Input: dimensioned drawing with shaded views. Units: mm. Origin: part minimum x, y, z. A direction names the side the tool comes from. Round coordinates to 2 decimals unless told otherwise and drop trailing zeros. Loops run counter-clockwise (first coordinate to the right, second up) from the corner with the lowest first, then second, coordinate; pieces in that order, holes last. Notation, with made-up numbers: (59, 1) - (102, 1) arc R29 ccw to (102, 40) - close; hole circle Ø10 at (72.5, 7). An arc over 180 degrees is marked (long way). Use CSV: the item, a comma, the result in double quotes. Start each with the question number.
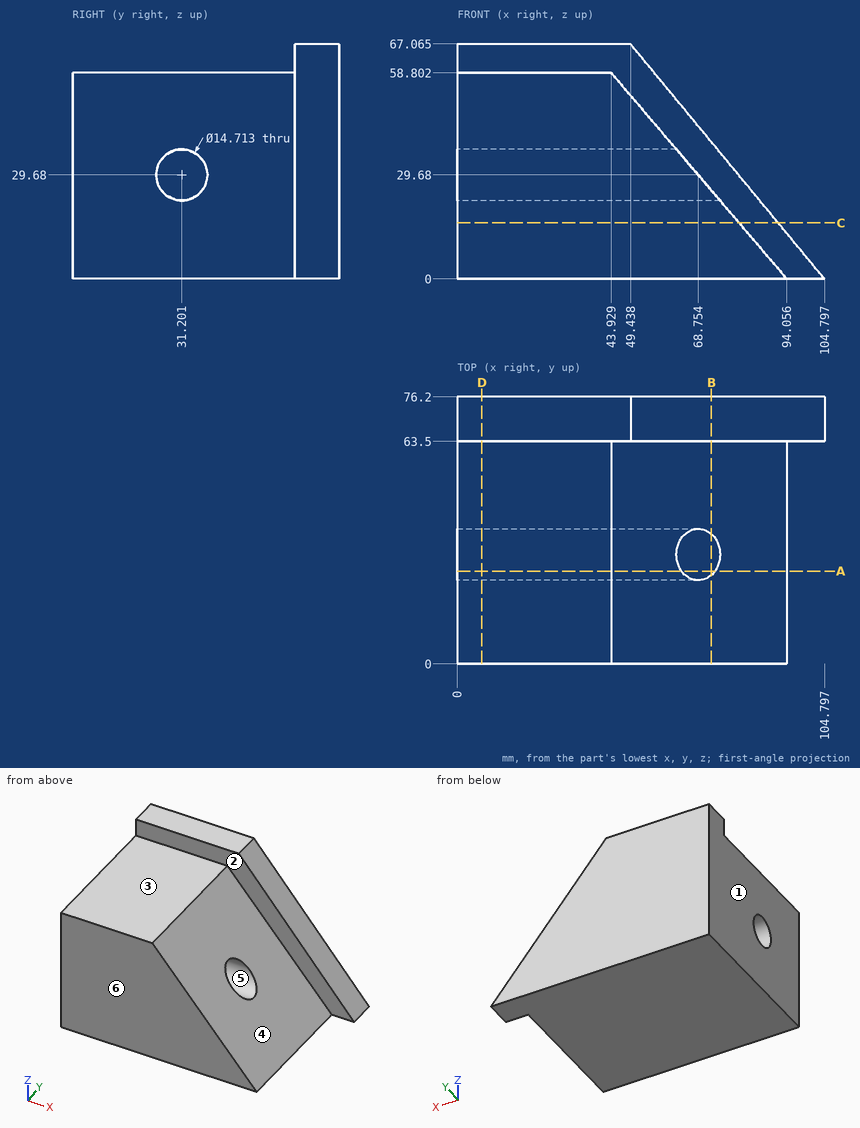
1. Section query D-D on x = 7. Return the cut outline in (y, z) (1 decimal).
2. Contact query for flat-ended pins moving along their axis: P1, Ø12, axis at x = 54.5, z = 59, coming from the -Y side; P2, Ø10, axis at x = 88, y = 29.5, coming from the +Z side. Output: stop coordinate, or through.
3. Line query: line 1 along Y through (x, z) = (69, 28); line 2 along Z through (x, y) = (55.5, 31) (1 decimal); line 3 along Y through (x, z) = (79.5, 30). Output: solid intervals per line, ascending.
4. Mould query, pull axis Y, two halves, no side actions, for the marked faces 4, 5 and 6. Classes: +Y half, -Y half, draft (parallel to the pull), parting line (faces both ways), or undercut.
5. Section query A-A on y = 26.5. Return the cut outline in (x, z) (1 decimal).
6. Reachability of the marked faces 1, 2 and 3 from +Z, -Z, +X, -X, +Y, -Y: full face, straight path, thin tool, end or side. Return the list, or none.
7. Section query C-C on z = 16. Return the cut outline in (x, y), and give its area (3 significant figures).
8. Section query B-B on x = 72.5. Return the cut outline in (y, z) (1 decimal), and give its area (3 significant figures).
Values:
1,outline,"(0, 0) - (76.2, 0) - (76.2, 67.1) - (63.5, 67.1) - (63.5, 58.8) - (0, 58.8) - close; hole circle Ø14.7 at (31.2, 29.7)"
2,P1,"stops at y = 63.5"
2,P2,"stops at z = 12.97"
3,line 1,"y = 0 to 24.04, 38.36 to 76.2"
3,line 2,"z = 0 to 22.3, 37 to 45.2"
3,line 3,"y = 63.5 to 76.2"
4,face 4,"draft"
4,face 5,"undercut"
4,face 6,"-Y half"
5,outline,"(0, 0) - (94.1, 0) - (73.6, 24) - (0, 24) - close; (0, 35.3) - (63.9, 35.3) - (43.9, 58.8) - (0, 58.8) - close"
6,face 1,"+Z, -Z, -X, +Y, -Y"
6,face 2,"+Z, +X, -Y"
6,face 3,"+Z, +X, -X, -Y"
7,outline,"(0, 0) - (80.42, 0) - (80.42, 63.5) - (91.59, 63.5) - (91.59, 76.2) - (0, 76.2) - close"
7,area,"6,270 mm^2"
8,outline,"(0, 0) - (76.2, 0) - (76.2, 39.1) - (63.5, 39.1) - (63.5, 25.3) - (37.1, 25.3) arc R7.4 cw to (25.3, 25.3) - (0, 25.3) - close"
8,area,"2,080 mm^2"
